```python
from build123d import *

# Parameters (mm, degrees)
SKETCH1_W                           = 389
SKETCH1_H                           = 39.998298848
SKETCH1_R                           = 10.5
SKETCH1_R_2                         = 6.35
MAIN_BODY_DEPTH                     = 30
Z_START                             = 16
SKETCH1_4_R                         = 10.25
SKETCH1_4_R_2                       = 6.35
Z_NUT_FLANGE_RECESS_DEPTH           = 20
SKETCH2_R                           = 1.25
LINEAR_BEARINGS_M3_PILOTS_DEPTH     = 5
SKETCH3_R                           = 6.35
Z_NUT_SCREW_THROUGH_HOLE_DEPTH      = 30
STEPPER_CUT_REACH                   = 403.624
SKETCH4_W                           = 250
SKETCH4_H                           = 21
M3_TAPPED_HOLE1_D                   = 2.5
M3_TAPPED_HOLE1_DEPTH               = 8.5
M3_TAPPED_HOLE1_TIP                 = 0.751075774
Z_NUT_SCREW_CLEARENCE_REACH         = 403.904
Z_NUT_SCREW_CLEARENCE_PATTERN_COUNT = 3
INSERT_THROUGH_HOLE_LOWER_G_REACH   = 403.904
SKETCH13_R                          = 5
CABLE_START                         = -16
SKETCH15_R                          = 1.25
CABLE_CLIPS_M3_PILOTS_DEPTH         = 418.904345655
M3_TAPPED_HOLE2_D                   = 2.5


with BuildPart() as part:
    # Sketch1 → Main Body (new body)
    with BuildSketch(Plane.XY):
        with Locations((-204, -22.719149424)):
            Rectangle(SKETCH1_W, SKETCH1_H)
        with Locations((-380.5, -21.75)):
            Circle(SKETCH1_R, mode=Mode.SUBTRACT)
        with Locations((-27.5, -21.75)):
            Circle(SKETCH1_R, mode=Mode.SUBTRACT)
        with Locations((-204, -27.1)):
            Circle(SKETCH1_R_2, mode=Mode.SUBTRACT)
    extrude(amount=MAIN_BODY_DEPTH)

    # Sketch1<4> → Z Nut Flange Recess (cut)
    with BuildSketch(Plane.XY.offset(Z_START)):
        with Locations((-204, -27.1)):
            Circle(SKETCH1_4_R)
        with Locations((-204, -27.1)):
            Circle(SKETCH1_4_R_2, mode=Mode.SUBTRACT)
        with Locations((-204, -27.1)):
            Circle(SKETCH1_4_R_2)
    extrude(amount=Z_NUT_FLANGE_RECESS_DEPTH, mode=Mode.SUBTRACT)

    # Sketch2 → Linear Bearings - M3 Pilots (cut)
    with BuildSketch(Plane(origin=(0, 0, 0), x_dir=(-1, 0, 0), z_dir=(0, 0, -1))):
        with Locations((16.186291501, -10.436291501)):
            Circle(SKETCH2_R)
        with Locations((38.813708499, -10.436291501)):
            Circle(SKETCH2_R)
        with Locations((16.186291501, -33.063708499)):
            Circle(SKETCH2_R)
        with Locations((38.813708499, -33.063708499)):
            Circle(SKETCH2_R)
        with Locations((369.186291501, -10.436291501)):
            Circle(SKETCH2_R)
        with Locations((391.813708499, -10.436291501)):
            Circle(SKETCH2_R)
        with Locations((369.186291501, -33.063708499)):
            Circle(SKETCH2_R)
        with Locations((391.813708499, -33.063708499)):
            Circle(SKETCH2_R)
    extrude(amount=-LINEAR_BEARINGS_M3_PILOTS_DEPTH, mode=Mode.SUBTRACT)

    # Sketch3 → Z Nut - Screw Through Hole (cut)
    with BuildSketch(Plane(origin=(0, 0, 0), x_dir=(-1, 0, 0), z_dir=(0, 0, -1))):
        with BuildLine():
            Line((205.55, -35.15), (205.55, -33.360990337))
            ThreePointArc((205.55, -33.360990337), (209.585863854, -30.325), (210.197176685, -25.311844207))
            Line((210.197176685, -25.311844207), (211.7465045, -24.417339376))
            ThreePointArc((211.7465045, -24.417339376), (212.313843876, -22.3), (210.1965045, -21.732660624))
            Line((210.1965045, -21.732660624), (208.647176685, -22.627165456))
            ThreePointArc((208.647176685, -22.627165456), (204, -20.65), (199.352823315, -22.627165456))
            Line((199.352823315, -22.627165456), (197.8034955, -21.732660624))
            ThreePointArc((197.8034955, -21.732660624), (195.686156124, -22.3), (196.2534955, -24.417339376))
            Line((196.2534955, -24.417339376), (197.802823315, -25.311844207))
            ThreePointArc((197.802823315, -25.311844207), (198.414136146, -30.325), (202.45, -33.360990337))
            Line((202.45, -33.360990337), (202.45, -35.15))
            ThreePointArc((202.45, -35.15), (204, -36.7), (205.55, -35.15))
        make_face()
        with Locations((204, -27.1)):
            Circle(SKETCH3_R, mode=Mode.SUBTRACT)
    extrude(amount=-Z_NUT_SCREW_THROUGH_HOLE_DEPTH, mode=Mode.SUBTRACT)

    # Sketch4 → Stepper Cut (cut, up to next)
    with BuildSketch(Plane(origin=(0, -2.72, 0), x_dir=(1, 0, 0), z_dir=(0, 1, 0)), mode=Mode.PRIVATE) as stepper_cut_sk1:
        with Locations((-204, -26.5)):
            Rectangle(SKETCH4_W, SKETCH4_H)
    stepper_cut_tool1 = extrude(stepper_cut_sk1.sketch, amount=-STEPPER_CUT_REACH, mode=Mode.PRIVATE) & part.part
    add(stepper_cut_tool1.solids().sort_by_distance((-204, -2.72, 26.5))[0], mode=Mode.SUBTRACT)

    # M3 Tapped Hole1
    with Locations(Plane(origin=(-16.186291501, -33.063708499, 0), x_dir=(-1, 0, 0), z_dir=(0, 0, -1))):
        with Locations((0, 0), (22.627416998, 0), (22.627416998, 22.627416998), (0, 22.627416998), (375.627416998, 22.627416998), (353, 22.627416998), (353, 0), (375.627416998, 0)):
            Hole(M3_TAPPED_HOLE1_D / 2, depth=M3_TAPPED_HOLE1_DEPTH)
            with Locations((0, 0, -(M3_TAPPED_HOLE1_DEPTH + M3_TAPPED_HOLE1_TIP / 2))):  # 118° drill point
                Cone(0, M3_TAPPED_HOLE1_D / 2, M3_TAPPED_HOLE1_TIP, mode=Mode.SUBTRACT)

    # Sketch12 → Z Nut Screw Clearence (cut, up to next)
    with BuildSketch(Plane(origin=(0, 0, 0), x_dir=(-1, 0, 0), z_dir=(0, 0, -1)), mode=Mode.PRIVATE) as z_nut_screw_clearence_sk1:
        with BuildLine():
            Line((205.75, -36.4), (205.75, -33.308059278))
            ThreePointArc((205.75, -33.308059278), (205.650212236, -33.335326742), (205.55, -33.360990337))
            Line((205.55, -33.360990337), (205.55, -35.15))
            ThreePointArc((205.55, -35.15), (204, -36.7), (202.45, -35.15))
            Line((202.45, -35.15), (202.45, -33.360990337))
            ThreePointArc((202.45, -33.360990337), (202.349787764, -33.335326742), (202.25, -33.308059278))
            Line((202.25, -33.308059278), (202.25, -36.4))
            ThreePointArc((202.25, -36.4), (204, -38.15), (205.75, -36.4))
        make_face()
    z_nut_screw_clearence_tool1 = extrude(z_nut_screw_clearence_sk1.sketch, amount=-Z_NUT_SCREW_CLEARENCE_REACH, mode=Mode.PRIVATE) & part.part
    z_nut_screw_clearence = z_nut_screw_clearence_tool1.solids().sort_by_distance((-202.309745, -34.85403, 0))[0]
    add(z_nut_screw_clearence, mode=Mode.SUBTRACT)

    # Z Nut Screw Clearence Pattern: Z Nut Screw Clearence ×3 about axis
    z_nut_screw_clearence_pattern_axis = Axis((-204, -27.1, 0), (0, 0, 1))
    for i in range(1, Z_NUT_SCREW_CLEARENCE_PATTERN_COUNT):
        add(z_nut_screw_clearence.rotate(z_nut_screw_clearence_pattern_axis, i * 360 / Z_NUT_SCREW_CLEARENCE_PATTERN_COUNT), mode=Mode.SUBTRACT)

    # Sketch13 → Insert Through Hole - Lower G (cut, up to next)
    with BuildSketch(Plane(origin=(0, 0, 0), x_dir=(-1, 0, 0), z_dir=(0, 0, -1)), mode=Mode.PRIVATE) as insert_through_hole_lower_g_sk1:
        with Locations((115.4, -22)):
            Circle(SKETCH13_R)
    insert_through_hole_lower_g_tool1 = extrude(insert_through_hole_lower_g_sk1.sketch, amount=-INSERT_THROUGH_HOLE_LOWER_G_REACH, mode=Mode.PRIVATE) & part.part
    # Sketch13 → Insert Through Hole - Lower G (cut, up to next)
    with BuildSketch(Plane(origin=(0, 0, 0), x_dir=(-1, 0, 0), z_dir=(0, 0, -1)), mode=Mode.PRIVATE) as insert_through_hole_lower_g_sk2:
        with Locations((322.6, -22)):
            Circle(SKETCH13_R)
    insert_through_hole_lower_g_tool2 = extrude(insert_through_hole_lower_g_sk2.sketch, amount=-INSERT_THROUGH_HOLE_LOWER_G_REACH, mode=Mode.PRIVATE) & part.part
    add(insert_through_hole_lower_g_tool1.solids().sort_by_distance((-115.4, -22, 0))[0], mode=Mode.SUBTRACT)
    add(insert_through_hole_lower_g_tool2.solids().sort_by_distance((-322.6, -22, 0))[0], mode=Mode.SUBTRACT)

    # Sketch15 → Cable Clips - M3 Pilots (cut, through all)
    with BuildSketch(Plane(origin=(0, 0, 0), x_dir=(-1, 0, 0), z_dir=(0, 0, -1)).offset(CABLE_START)):
        with Locations(Location((154, -22.719149424, 0), (0, 0, 180))):
            Circle(SKETCH15_R)
        with Locations(Location((254, -22.719149424, 0), (0, 0, 180))):
            Circle(SKETCH15_R)
    extrude(amount=CABLE_CLIPS_M3_PILOTS_DEPTH, mode=Mode.SUBTRACT)

    # M3 Tapped Hole2 (through all)
    with Locations(Plane(origin=(-154, -22.719149424, 16), x_dir=(1, 0, 0), z_dir=(0, 0, 1))):
        with Locations((0, 0), (-100, 0)):
            Hole(M3_TAPPED_HOLE2_D / 2)


solid = part.part
```
Input: part model. Units: mm. Frame: model coordinates. A direction names the side the tool comes from. Give positions to 0.01 mm unless a question says otherwise; leave off trailing zeros. Write each loop counter-clockwise with the first axis right and the second up, starting at its lowest first coordinate (ties: lowest second). Pieces come first, ordered by that corner, then holes. Notation, with made-up numbers: (74.5, -24) - (100.5, -24) arc R23 cw to (100.5, -4) - close; hole circle Ø2 at (63.5, 23.5). An arc over 180 degrees is marked (long way). Write item = value, one per line. Start each with the question number.
1. Access query for faces 1 (the cylindrical face through (-198.4, -30.3, 7.9)), 2 (the flat face through (-364, -22, 30)), 3 (the flat face through (-79, -22, 23)). Directions: +Z, -Z, +X, -X, +Y, -Y. A direction counts if a zero-diameter tool reaches every point of the face in a straight line with its end or side. Return the directions, or none.
2. First-contact query: pin 1 Ø12 at (x, y) = (-203, -16) entering from +Z; pin 2 Ø2 at (x, y) = (-369.19, -33.06) entering from -Z; pin 3 Ø3 at (x, y) = (-254, -22.72) entering from -Z. Flat tips, straight axial feed; report the tip coordinate or a pass-through.
3. Section query B-B, the plane x = -322.6. Output: boundary loops of the cut face in (y, z).
4. Section query D-D, the plane x = -97. Output: boundary loops of the cut face in (y, z).
5. Section query A-A, the plane z = 26.75. Output: boundary loops of the cut face in (x, y).
6. Ray query, L1, parallel to X at y = -22, z = 21; L2, parallel to X at y = -11, z = 24; L3, parallel to Y at x = -154, z = 11. Return the intervals inside material, ascending.
7. Section query C-C, the plane x = -27.5. Output: boundary loops of the cut face in (y, z).
8. Mould query, pull axis X, two halves, no side actions, for faces 4 (the flat face through (-398.5, -23, 15)), 5 (the cylindrical face through (-209.55, -30.39, 7.89)), 6 (the flat face through (-206, -18, 16)), 7 (the flat face through (-207, -2.72, 11)). Classes: released by +X, released by -X, zero draft, split by the parting line, or undercut.
Check sheet entries:
q1.face_1 = +Z, -Z
q1.face_2 = +Z, +X, -X, +Y, -Y
q1.face_3 = +Z, +Y, -Y
q2.pin_1 = 16
q2.pin_2 = 8.65
q2.pin_3 = 0
q3.outline = (-42.72, 0) - (-27, 0) - (-27, 16) - (-42.72, 16) - close; (-17, 0) - (-2.72, 0) - (-2.72, 16) - (-17, 16) - close
q4.outline = (-42.72, 0) - (-2.72, 0) - (-2.72, 16) - (-42.72, 16) - close
q5.outline = (-398.5, -42.72) - (-329, -42.72) - (-329, -2.72) - (-398.5, -2.72) - close; (-79, -42.72) - (-9.5, -42.72) - (-9.5, -2.72) - (-79, -2.72) - close; hole circle Ø21 at (-380.5, -21.75); hole circle Ø21 at (-27.5, -21.75)
q6.L1 = -398.5 to -391, -370 to -329, -79 to -38, -17 to -9.5
q6.L2 = -398.5 to -329, -79 to -9.5
q6.L3 = -42.72 to -23.97, -21.47 to -2.72
q7.outline = (-42.72, 0) - (-32.25, 0) - (-32.25, 30) - (-42.72, 30) - close; (-11.25, 0) - (-2.72, 0) - (-2.72, 30) - (-11.25, 30) - close
q8.face_4 = released by -X
q8.face_5 = undercut
q8.face_6 = undercut
q8.face_7 = zero draft
